Can you work these out from the drawing? Everything is in mm from the part's minimum corner. Coordinates: 2 decimals unless noted, no trailing zeros. Loops run counter-clockwise (first coordinate to the right, second up) from the corner with the lowest first, then second, coordinate; pieces in that order, holes last. Notation, with made-up numbers: (83.5, -6) - (126.5, -6) arc R20 ccw to (126.5, 32) - close; hole circle Ø10 at (26.25, -14). An arc over 180 degrees is marked (long way). Put each result on its own line as item: value. Start each with the question number.
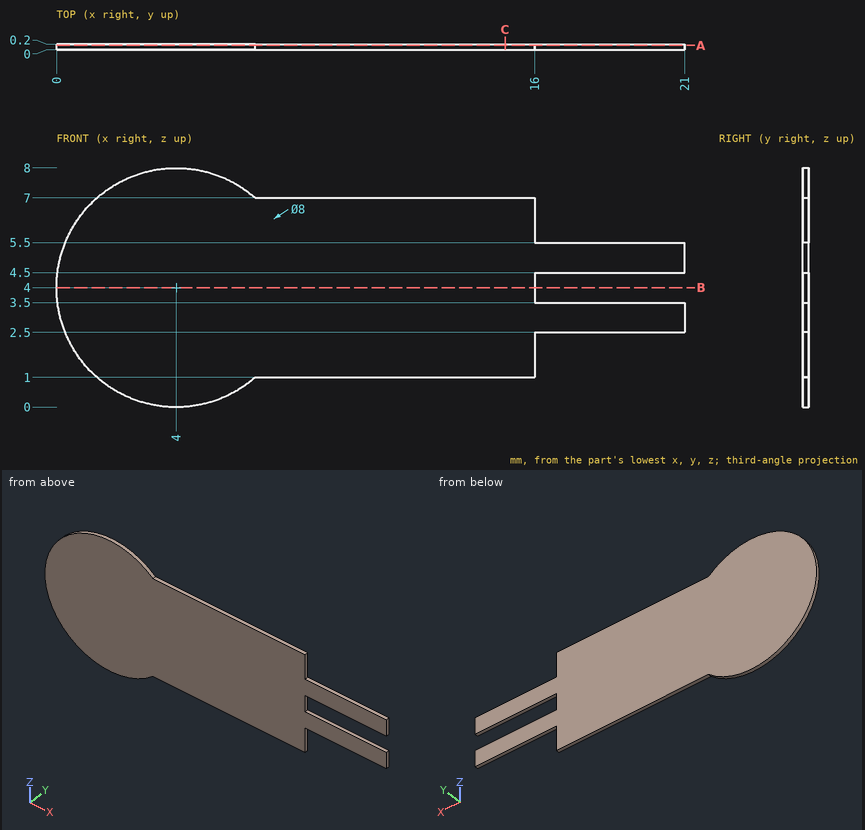
(1) I want a section at A-A on y = 0.15. List the corners of the cut face in (x, z) for me.
(2) I need wall thicknesses on L1, parallel to Z at x = 19.5, y = 0.1; L2, parallel to X at y = 0.1, z = 5.25; L3, parallel to Z at x = 8, y = 0.1. Which ranges of each line are inside material? Lowest first, please. Write a range as [from, to].
(3) I want a section at B-B on z = 4. List the corners of the cut face in (x, y) for me.
(4) I want a section at C-C on x = 15. List the corners of the cut face in (y, z) for me.
Answer sheet:
1. outline: (6.65, 1) - (16, 1) - (16, 2.5) - (21, 2.5) - (21, 3.5) - (16, 3.5) - (16, 4.5) - (21, 4.5) - (21, 5.5) - (16, 5.5) - (16, 7) - (6.65, 7) arc R4 ccw (long way) to start
2. L1: z = [2.5, 3.5], [4.5, 5.5]
2. L2: x = [0.2, 21]
2. L3: z = [1, 7]
3. outline: (0, 0) - (16, 0) - (16, 0.2) - (0, 0.2) - close
4. outline: (0, 1) - (0.2, 1) - (0.2, 7) - (0, 7) - close
